Answer from the drawing. Dimensions are ordinates in mm from the lowest x, y and z of the part. Coordinates: 2 decimals unless noted, no trailing zeros. Order: outer loops, then holes, each group sorted by start corner. A loop starts at its lowest first (then second) coordinate and runs counter-clockwise, first axis right, second up. Notation, with made-up numbers: M -36.5,54.25 L 22.5,54.25 A24 ccw 22.5,83.25 Z; hole C -26.75,43 d9. An arc over 180 degrees is marked long. Write each question's results on one line, items separated by ' | '.
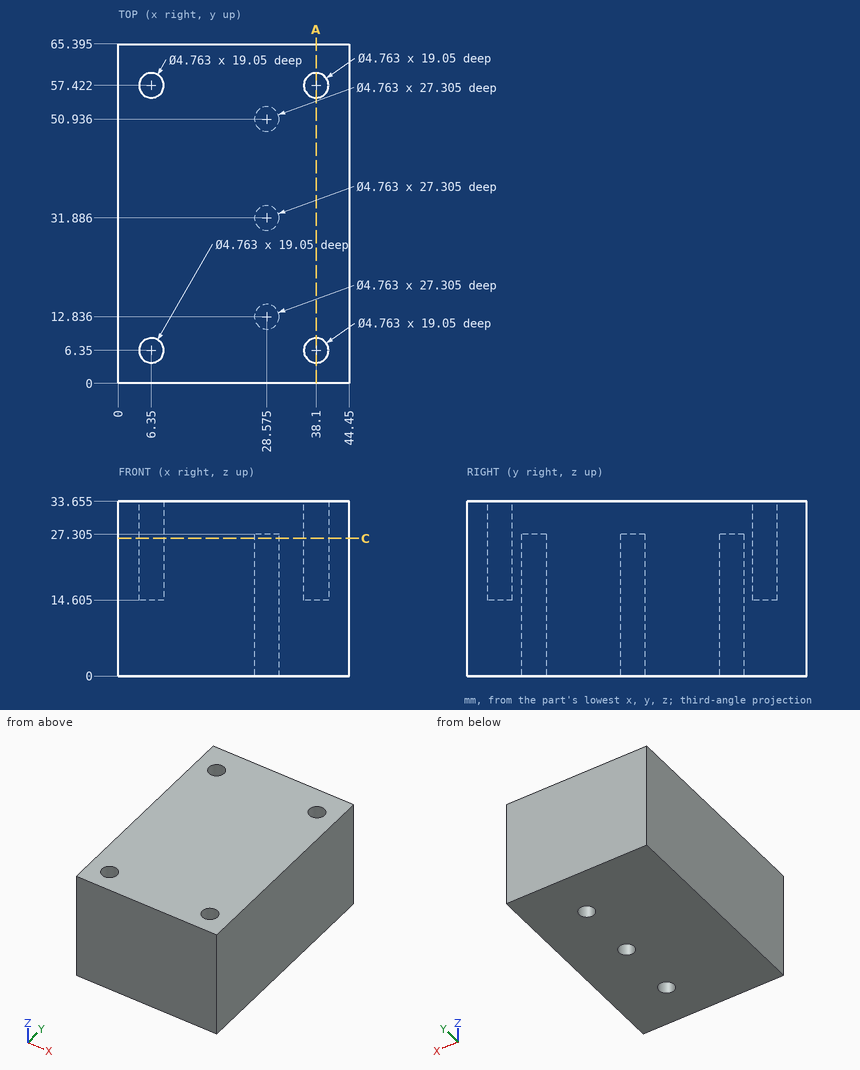
(1) Given pin 1 (2.5 mm diameter, centred on x = 29.5, y = 51, fed in from -Z) (3 decimals); pin 2 (1.4 mm diameter, centred on x = 38.5, y = 57, fed in from +Z) (3 decimals), each flat-ended and moving along its own axis, determine where each tip first touches the part or whether it passes through.
Conclusion:
pin 1: z = 27.305 | pin 2: z = 14.605
(2) Straight lines are drawn through the part: line 1 (Y direction, x = 38.1, z = 25.5) (1 decimal); line 2 (X direction, y = 5, z = 23.5); line 3 (X direction, y = 13, z = 8). For each, find the intervals that lie inside material, in ascending order.
Conclusion:
line 1: 0 to 4, 8.7 to 55, 59.8 to 65.4 | line 2: 0 to 4.39, 8.31 to 36.14, 40.06 to 44.45 | line 3: 0 to 26.2, 30.95 to 44.45
(3) The part is cut by section A-A, the plane x = 38.1. Write down the section's boundary in (y, z) (1 decimal), then the cut area to 3 significant figures.
Conclusion:
outline: M 0,0 L 65.4,0 L 65.4,33.7 L 59.8,33.7 L 59.8,14.6 L 55,14.6 L 55,33.7 L 8.7,33.7 L 8.7,14.6 L 4,14.6 L 4,33.7 L 0,33.7 Z | area: 2,020 mm²
(4) The part is cut by section C-C, the plane z = 26.5. Count the separate pieces of the cut face and the enclosed holes in it, then the cut area to 3 significant figures.
Conclusion:
separate pieces: 1 | enclosed holes: 7 | area: 2,780 mm²
